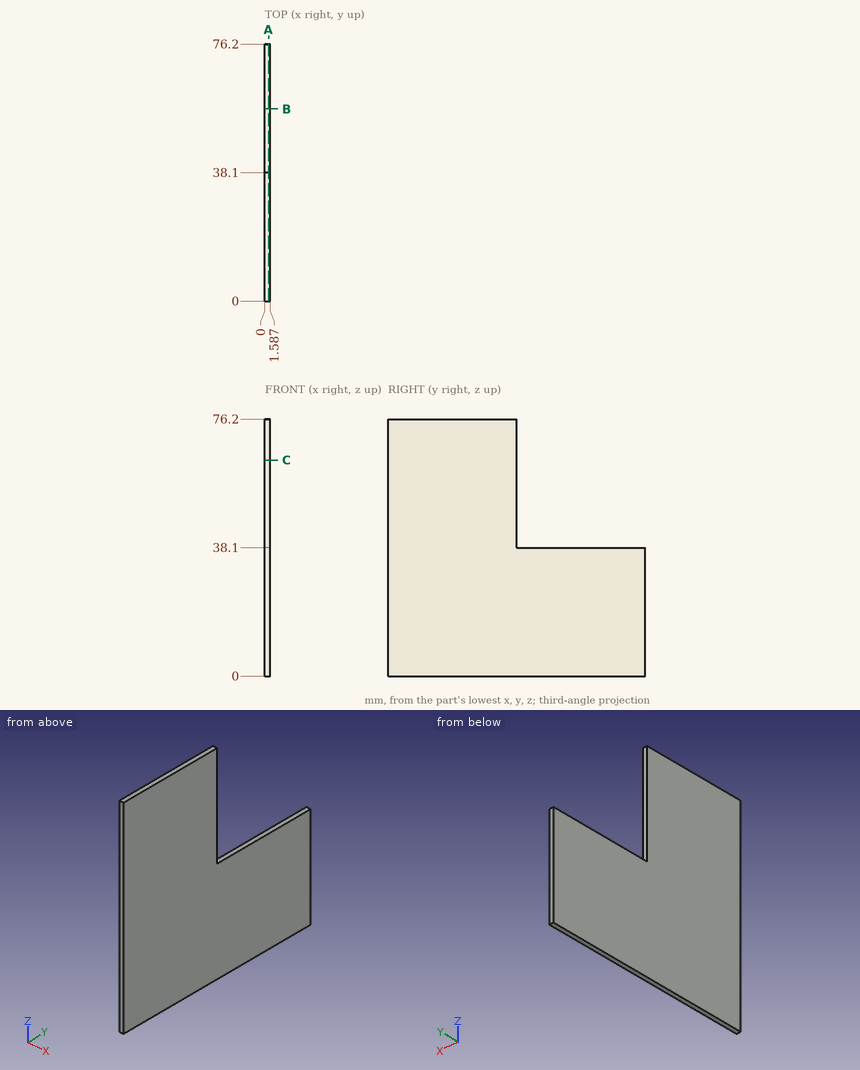
Input: dimensioned drawing with shaded views. Units: mm. Origin: part minimum x, y, z. Coordinates: 2 decimals unless noted, no trailing zeros. Write each loop counter-clockwise with the first axis right and the second up, starting at its lowest first coordinate (ties: lowest second). Pieces come first, ordered by that corner, then holes. Notation, with made-up numbers: M 49.25,63 L 107.25,63 A29 cw 107.25,94 Z; hole C 73,77.25 d9. An arc over 180 degrees is marked long. Use one line per item in the form item = value.
Q1. Section B-B (y = 57). Return loops of the section in (x, z).
Answer below:
outline = M 0,0 L 1.59,0 L 1.59,38.1 L 0,38.1 Z
Q2. Material intervals for probe 1 along Y at (x, z) = (0.15, 56), sorted ascending. Write a range as from..to.
Answer below:
probe_1 = 0..38.1
Q3. First-contact query: pin 1 (0.8 mm diameter, centred on x = 0.5, z = 57.5, fed in from +Y). Flat tip, straight axial feed; report the tip coordinate or a pass-through.
Answer below:
pin_1 = 38.1
Q4. Section A-A (x = 1.1). Return loops of the section in (y, z), plus the area to 4 significant figures.
Answer below:
outline = M 0,0 L 76.2,0 L 76.2,38.1 L 38.1,38.1 L 38.1,76.2 L 0,76.2 Z
area = 4,355 mm²
